Verification items for the finished model (mm, model axes). A direction names the side the tool comes from. Give positions to 0.01 mm unless a question says otherwise; leave off trailing zeros. Loops run counter-clockwise (first coordinate to the right, second up) from the corner with the lowest first, then second, coordinate; pieces in that order, holes last. Notation, with made-up numbers: (35.25, 52.25) - (71.25, 52.25) arc R22 ccw to (71.25, 65.25) - close; hole circle Ø7 at (-38.75, 32.5). An arc over 180 degrees is marked (long way). Answer in a Markdown table with one row per item.
```python
from build123d import *

# Parameters (mm, degrees)
SKETCH_1_W      = 64.5
SKETCH_1_H      = 39
SKETCH_1_W_2    = 62.5
SKETCH_1_H_2    = 37
EXTRUDE_2_DEPTH = 3
SKETCH_2_W      = 70
SKETCH_2_H      = 45
SKETCH_2_W_2    = 62.5
SKETCH_2_H_2    = 37
EXTRUDE_3_DEPTH = 15
SKETCH_4_W      = 70
SKETCH_4_H      = 1
EXTRUDE_4_DEPTH = 22.5
FILLET_1_R      = 5
FILLET_2_R      = 5


with BuildPart() as part:
    # 草图1 → 凸台-拉伸2 (new body)
    with BuildSketch(Plane(origin=(0, 0, 0), x_dir=(1, 0, 0), z_dir=(0, 1, 0))):
        Rectangle(SKETCH_1_W, SKETCH_1_H)
        Rectangle(SKETCH_1_W_2, SKETCH_1_H_2, mode=Mode.SUBTRACT)
    extrude(amount=EXTRUDE_2_DEPTH)

    # 草图2 → 凸台-拉伸3 (add)
    with BuildSketch(Plane(origin=(0, 0, 0), x_dir=(1, 0, 0), z_dir=(0, 1, 0))):
        Rectangle(SKETCH_2_W, SKETCH_2_H)
        Rectangle(SKETCH_2_W_2, SKETCH_2_H_2, mode=Mode.SUBTRACT)
    extrude(amount=-EXTRUDE_3_DEPTH)

    # 草图4 → 凸台-拉伸4 (add, symmetric)
    with BuildSketch(Plane.XY):
        with Locations((0, -15.5)):
            Rectangle(SKETCH_4_W, SKETCH_4_H)
    extrude(amount=EXTRUDE_4_DEPTH, both=True)

    # 圆角1
    fillet_1_edges = [part.edges().sort_by_distance(p)[0] for p in [
        (35, -8, -22.5),
        (35, -8, 22.5),
        (-35, -8, 22.5),
        (-35, -8, -22.5),
    ]]
    fillet(fillet_1_edges, radius=FILLET_1_R)

    # 圆角2
    fillet_2_edges = [part.edges().sort_by_distance(p)[0] for p in [
        (0, -16, 22.5),
        (35, -16, 0),
        (0, -16, -22.5),
        (-35, -16, 0),
        (-33.535533906, -16, -21.035533906),
        (-33.535533906, -16, 21.035533906),
        (33.535533906, -16, -21.035533906),
        (33.535533906, -16, 21.035533906),
    ]]
    fillet(fillet_2_edges, radius=FILLET_2_R)


solid = part.part
```
Q1. Sectioned sample at A-A (y = -5). Record the cut outline in (x, z), and give its area (3 significant figures).
Completed:
| item | result |
|---|---|
| outline | (-35, -17.5) arc R5 ccw to (-30, -22.5) - (30, -22.5) arc R5 ccw to (35, -17.5) - (35, 17.5) arc R5 ccw to (30, 22.5) - (-30, 22.5) arc R5 ccw to (-35, 17.5) - close; hole (-31.25, -18.5) - (31.25, -18.5) - (31.25, 18.5) - (-31.25, 18.5) - close |
| area | 816 mm^2 |
Q2. Sectioned sample at B-B (x = -16). Record the cut outline in (y, z).
Completed:
| item | result |
|---|---|
| outline | (-16, -17.5) arc R5 ccw to (-11, -22.5) - (0, -22.5) - (0, -19.5) - (3, -19.5) - (3, -18.5) - (-15, -18.5) - (-15, 18.5) - (3, 18.5) - (3, 19.5) - (0, 19.5) - (0, 22.5) - (-11, 22.5) arc R5 ccw to (-16, 17.5) - close |
Q3. Go/stop test with flat-tipped pins: P1, Ø11, axis at x = 3.5, z = 4, coming from the +Y side; P2, Ø1.5, axis at x = 9, y = 1, coming from the +Z side; P3, Ø0.9, axis at x = 5.5, y = 2, coming from the -Z side. Record where each tip stops, or that it passes through.
Completed:
| item | result |
|---|---|
| P1 | y = -15 |
| P2 | z = 19.5 |
| P3 | z = -19.5 |
Q4. Thickness scan on line 1 (Z direction, x = -16, y = -1.5); line 2 (X direction, y = -3.5, z = 8); line 3 (Z direction, x = 4.5, y = 1.5). Record the ranges inside material, lowest first.
Completed:
| item | result |
|---|---|
| line 1 | -22.5 to -18.5, 18.5 to 22.5 |
| line 2 | -35 to -31.25, 31.25 to 35 |
| line 3 | -19.5 to -18.5, 18.5 to 19.5 |
Q5. Sectioned sample at C-C (z = -10). Record the cut outline in (x, y).
Completed:
| item | result |
|---|---|
| outline | (-35, -11) arc R5 ccw to (-30, -16) - (30, -16) arc R5 ccw to (35, -11) - (35, 0) - (32.25, 0) - (32.25, 3) - (31.25, 3) - (31.25, -15) - (-31.25, -15) - (-31.25, 3) - (-32.25, 3) - (-32.25, 0) - (-35, 0) - close |
Q6. Sectioned sample at D-D (y = -14.25). Record the cut outline in (x, z), and give its area (3 significant figures).
Completed:
| item | result |
|---|---|
| outline | (-33.8, -17.5) arc R3.8 ccw to (-30, -21.3) - (30, -21.3) arc R3.8 ccw to (33.8, -17.5) - (33.8, 17.5) arc R3.8 ccw to (30, 21.3) - (-30, 21.3) arc R3.8 ccw to (-33.8, 17.5) - close; hole (-31.25, -18.5) - (31.25, -18.5) - (31.25, 18.5) - (-31.25, 18.5) - close |
| area | 555 mm^2 |
Q7. Tool access check on faces 4 (the face through (-32.25, 1, 0)), 5 (the face through (0, 1, 19.5)), 6 (the face through (0, -15, 0)), 7 (the face through (0, 1, -19.5)). Record the directions out of +Z, -Z, +X, -X, +Y, -Y that give a thin tool (end or side, any length) a straight path to the whole face; none if there is none.
Completed:
| item | result |
|---|---|
| face 4 | +Z, -Z, -X, +Y |
| face 5 | +Z, +X, -X, +Y |
| face 6 | +Y |
| face 7 | -Z, +X, -X, +Y |
Q8. Draft check along X on faces 1 (the face through (32.25, 1, 0)), 2 (the face through (0, -6, -18.5)), 3 (the face through (0, -5, -22.5)). Enter one of: +X half, -X half, draft (parallel to the pull), parting line (faces both ways), or undercut.
Completed:
| item | result |
|---|---|
| face 1 | +X half |
| face 2 | undercut |
| face 3 | draft |
